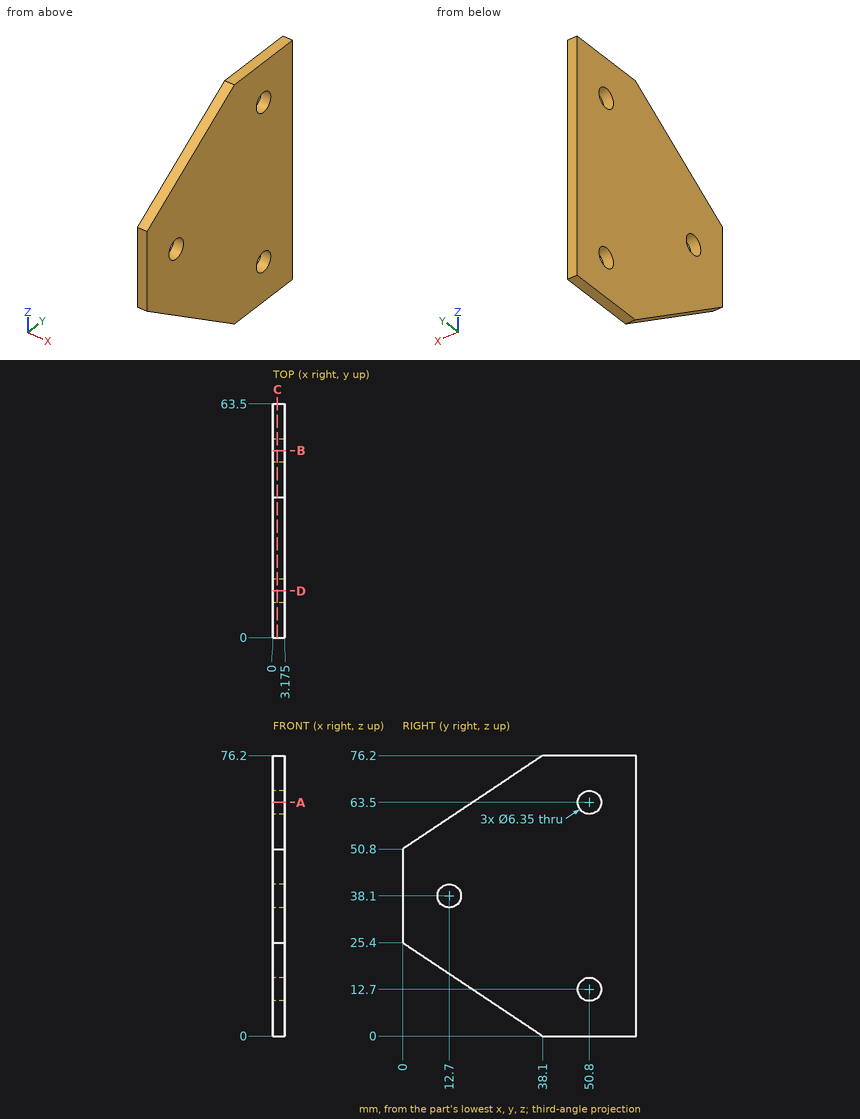
Input: dimensioned drawing with shaded views. Units: mm. Origin: part minimum x, y, z. Coordinates: 2 decimals unless noted, no trailing zeros. Write each loop counter-clockwise with the first axis right and the second up, starting at its lowest first coordinate (ties: lowest second). Pieces come first, ordered by that corner, then holes. Notation, with made-up numbers: M -31,-32.75 L 12,-32.75 A17 cw 12,-3.75 Z; hole C 54,76 d1. An arc over 180 degrees is marked long. Use one line per item in the form item = value.
Q1. Section B-B (y = 50.8). Return loops of the section in (x, z) (3 decimals).
Answer below:
outline = M 0,0 L 3.175,0 L 3.175,9.525 L 0,9.525 Z; M 0,15.875 L 3.175,15.875 L 3.175,60.325 L 0,60.325 Z; M 0,66.675 L 3.175,66.675 L 3.175,76.2 L 0,76.2 Z
Q2. First-contact query: pin 1 (4 mm diameter, centred on y = 16.5, z = 52, fed in from -X). Flat tip, straight axial feed; report the tip coordinate or a pass-through.
Answer below:
pin_1 = 0
Q3. Section C-C (x = 1.2). Return loops of the section in (y, z) (3 decimals), plus the area to 3 significant figures.
Answer below:
outline = M 0,25.4 L 38.1,0 L 63.5,0 L 63.5,76.2 L 38.1,76.2 L 0,50.8 Z; hole C 12.7,38.1 d6.35; hole C 50.8,12.7 d6.35; hole C 50.8,63.5 d6.35
area = 3,780 mm²
Q4. Section D-D (y = 12.7). Return loops of the section in (x, z) (3 decimals).
Answer below:
outline = M 0,16.933 L 3.175,16.933 L 3.175,34.925 L 0,34.925 Z; M 0,41.275 L 3.175,41.275 L 3.175,59.267 L 0,59.267 Z
Q5. Material intervals for probe 1 along Z at (x, y) = (0.8, 50.8) (3 decimals); probe 2 along Z at (x, y) = (1.5, 52.5); probe 3 along Y at (x, z) = (1.2, 38.1) (3 decimals), sorted ascending. Write a range as from..to.
Answer below:
probe_1 = 0..9.525, 15.875..60.325, 66.675..76.2
probe_2 = 0..10.02, 15.38..60.82, 66.18..76.2
probe_3 = 0..9.525, 15.875..63.5
Q6. Section A-A (z = 63.5). Return loops of the section in (x, y) (3 decimals).
Answer below:
outline = M 0,19.05 L 3.175,19.05 L 3.175,47.625 L 0,47.625 Z; M 0,53.975 L 3.175,53.975 L 3.175,63.5 L 0,63.5 Z
